The model under review builds one solid part; all positions refer to its coordinate system, in mm. A direction names the side the tool comes from. Coordinates: 2 decimals unless noted, no trailing zeros. Order: outer loops, then holes, each group sorted by start corner. A loop starts at its lowest first (then second) coordinate and runs counter-clockwise, first axis right, second up. Notation, with made-up numbers: M 39.25,-10.75 L 60.25,-10.75 A7 cw 60.25,2.25 Z; hole C 4.5,7 d1. An arc over 180 degrees is marked long. Answer as CSV lines item,"result". Start each with the question number.
Q1. For P1, Ø16, axis at y = 13.5, z = -11, coming from the +X side; P2, Ø1.5, axis at x = -32.5, y = 44.5, coming from the -Z side; P3, Ø16, axis at y = 9, z = -11.5, coming from the -X side; P4, Ø10, axis at x = 2, z = -15.5, coming from the +Y side, all flat-tipped, find the tip position at first contact; note any pin that passes through.
Q2. Consider section B-B on y = 11. Write out the cut boundary in (x, z).
Q3. Consider section A-A on x = 19.5. Write out the cut boundary in (y, z), and give its area (3 significant figures).
Q4. Machinability: for faces 1 (the face through (30, 1.8, -9.3)), 2 (the face through (-30, 1, -8)), 3 (the face through (0, 2, -15)), which of the approach directions +Z, -Z, +X, -X, +Y, -Y give a long, thin tool a straight path to every point of the face, cutting with its end or side? Answer none if there is none.
Q5. Wall thickness on L1, parallel to Z at x = 50, y = 41: over which ranges is the line inside the solid? List them lowest first. Write a range as [from, to].
Autodesk Inventor part; units mm, degrees
ref_plane "YZ Plane" through (0, 0, 0) normal (1, 0, 0) x (0, 1, 0)
ref_plane "XZ Plane" through (0, 0, 0) normal (0, 1, 0) x (-1, 0, 0)
ref_plane "XY Plane" through (0, 0, 0) normal (0, 0, 1) x (1, 0, 0)
sketch "Sketch1" plane through (0, 0, 0) normal (0, 0, 1) x (1, 0, 0)
  line L0 (60, 40) -> (60, 110)
  line L1 (60, 110) -> (-60, 110)
  line L2 (-60, 110) -> (-60, 40)
  line L3 (-30, 0) -> (30, 0)
  line L4 (30, 0) -> (30, 20)
  line L5 (-30, 20) -> (-30, 0)
  line L6 (-60, 40) -> (-30, 20)
  line L7 (30, 20) -> (60, 40)
  point P0 (0, 0)
  dimension "d4" = 120
  dimension "d5" = 70
  dimension "d7" = 20
  dimension "d8" = 60
extrude "Extrusion1" add sketch "Sketch1" along normal blind 2
sketch "Sketch2" plane through (-30, 0, 0) normal (0, -1, 0) x (1, 0, 0)
  line L0 (60, 0) -> (60, 2)
  line L1 (60, 0) -> (0, 0)
  line L2 (0, 0) -> (0, -30)
  line L3 (0, -30) -> (60, -30)
  line L4 (60, -30) -> (60, 0)
  dimension "d11" = 60
  dimension "d12" = 30
extrude "Extrusion2" add sketch "Sketch2" against normal blind 2
properties part number "Body Back"
Evaluation:
1,P1,"passes through"
1,P2,"stops at z = 0"
1,P3,"stops at x = -30"
1,P4,"stops at y = 2"
2,outline,"M -30,0 L 30,0 L 30,2 L -30,2 Z"
3,outline,"M 0,-30 L 2,-30 L 2,0 L 110,0 L 110,2 L 0,2 Z"
3,area,"280 mm²"
4,face 1,"+Z, -Z, +X, -Y"
4,face 2,"+Z, -Z, -X, -Y"
4,face 3,"-Z, +X, -X, +Y"
5,L1,"z = [0, 2]"
